```python
from build123d import *

# Parameters (mm, degrees)
F0_W      = 75
F0_H      = 75
F1_DEPTH  = 5
F3_DEPTH  = 40
F4_W      = 18
F4_H      = 17.9855290949
F4_W_2    = 12
F4_H_2    = 12
F4_H_3    = 18
F5_DEPTH  = 5
F6_DEPTH  = 15
F7_W      = 12
F7_H      = 15
F8_DEPTH  = 5
F9_W      = 12
F9_H      = 15
F10_DEPTH = 5


with BuildPart() as f1:
    # F0 (on Top) → F1 (new body)
    with BuildSketch(Plane.XY):
        Rectangle(F0_W, F0_H)
    extrude(amount=F1_DEPTH)

    # F2 (on face) → F3 (join)
    with BuildSketch(Plane.XY.offset(5)):
        Polygon((18.3847763109, 0), (0, 18.3847763109), (-18.3847763109, 0), (0, -18.3847763109), align=None)
        Polygon((-14.1421356237, 0), (0, 14.1421356237), (14.1421356237, 0), (0, -14.1421356237), align=None, mode=Mode.SUBTRACT)
    extrude(amount=F3_DEPTH)

    # F4 (on face) → F5 (join)
    with BuildSketch(Plane.XY.offset(5)):
        with Locations((0.0273990361, 28.5072354525)):
            Rectangle(F4_W, F4_H)
        with Locations((0.0273990361, 28.5144709051)):
            Rectangle(F4_W_2, F4_H_2, mode=Mode.SUBTRACT)
        with Locations((-28.5, 0)):
            Rectangle(F4_W, F4_H_3)
        with Locations((-28.5, 0)):
            Rectangle(F4_W_2, F4_H_2, mode=Mode.SUBTRACT)
    extrude(amount=F5_DEPTH)

    # F6 (add): faces of the model
    f6_faces = [f1.faces().sort_by_distance(p)[0] for p in [
        (8.772942899, 28.5072354525, 10),
        (-28.5, 8.7454415588, 10),
        (-28.5, 8.7454415588, 10),
    ]]
    extrude(f6_faces, amount=F6_DEPTH)

    # F7 (on face) → F8 (cut)
    with BuildSketch(Plane(origin=(-37.5, 0, 0), x_dir=(0, -1, 0), z_dir=(-1, 0, 0))):
        with Locations((0, 17.5)):
            Rectangle(F7_W, F7_H)
    extrude(amount=-F8_DEPTH, mode=Mode.SUBTRACT)

    # F9 (on face) → F10 (cut)
    with BuildSketch(Plane(origin=(0, 37.5, 0), x_dir=(-1, 0, 0), z_dir=(0, 1, 0))):
        with Locations((0, 17.5)):
            Rectangle(F9_W, F9_H)
    extrude(amount=-F10_DEPTH, mode=Mode.SUBTRACT)


solid = f1.part
```
Geometry check sheet. Reference: the model listing, model coordinates, mm. A direction names the side the tool comes from. Give positions to 0.01 mm unless a question says otherwise; leave off trailing zeros. Loops run counter-clockwise (first coordinate to the right, second up) from the corner with the lowest first, then second, coordinate; pieces in that order, holes last. Notation, with made-up numbers: M -21.75,71.5 L 20.25,71.5 A13 ccw 20.25,79.5 Z; hole C 50,-25.75 d4. An arc over 180 degrees is marked long. Write item = value, one per line.
(1) Release check for a two-part mould opening along X. For faces 6 (the face through (-30, 6, 15)), 7 (the face through (-8.973, 28, 15)), 8 (the face through (9.321, 9.064, 24.72)), 9 (the face through (7.17, -6.97, 24.72)) record: released by +X, released by -X, zero draft, split by the parting line, or undercut.
Answer below:
face_6 = undercut
face_7 = released by -X
face_8 = released by +X
face_9 = undercut
(2) Material ranges on line 1 (X direction, y = 1, z = 20.5); line 2 (Y direction, x = -27.5, z = 24.5); line 3 (X direction, y = -5.5, z = 15), recorded low to high. Write a range as [from, to].
Answer below:
line_1 = [-22.5, -19.5], [-17.38, -13.14], [13.14, 17.38]
line_2 = [-9, -6], [6, 9]
line_3 = [-22.5, -19.5], [-12.88, -8.64], [8.64, 12.88]
(3) Sectioned sample at D-D, the plane x = -20.5. Record the cut outline in (y, z).
Answer below:
outline = M -37.5,0 L 37.5,0 L 37.5,5 L 9,5 L 9,25 L -9,25 L -9,5 L -37.5,5 Z
(4) Sectioned sample at A-A, the plane z = 11. State how many separate pieces and enclosed holes the cut face has, plus the area to 3 significant figures.
Answer below:
separate_pieces = 3
enclosed_holes = 1
area = 564 mm2
(5) Gauge pin test, flat ends, axial feed: pin 1 Ø6 at (x, z) = (20, 27) entering from -Y; pin 2 Ø3 at (y, z) = (-7.5, 25.5) entering from +X; pin 3 Ø8 at (y, z) = (-14.5, 13) entering from -X; pin 4 Ø8 at (x, y) = (-25.5, 8.5) entering from -Z. Record the tip position at first contact, or that the pin passes through.
Answer below:
pin_1 = -1.38
pin_2 = 12.38
pin_3 = -7.88
pin_4 = 0
(6) Sectioned sample at B-B, the plane y = 30. Record the cut outline in (x, z), plus the area to 3 significant figures.
Answer below:
outline = M -37.5,0 L 37.5,0 L 37.5,5 L 9.03,5 L 9.03,25 L 6.03,25 L 6.03,5 L -5.97,5 L -5.97,25 L -8.97,25 L -8.97,5 L -37.5,5 Z
area = 495 mm2
(7) Sectioned sample at C-C, the plane z = 27.5. Record the cut outline in (x, y), plus the area to 3 significant figures.
Answer below:
outline = M -18.38,0 L 0,-18.38 L 18.38,0 L 0,18.38 Z; hole M -14.14,0 L 0,-14.14 L 14.14,0 L 0,14.14 Z
area = 276 mm2
(8) Tool access check on faces 1 (the face through (-7.17, 6.97, 24.72)), 2 (the face through (9.064, -9.321, 24.72)), 3 (the face through (-29, 9, 15)), 4 (the face through (6, 36, 17)), 5 (the face through (-21, 2, 25)). Record the directions out of +Z, -Z, +X, -X, +Y, -Y that give a thin tool (end or side, any length) a straight path to the whole face; none if there is none.
Answer below:
face_1 = +Z
face_2 = +Z, +X, -Y
face_3 = +Z, -X, +Y
face_4 = +Z, +Y
face_5 = +Z, -X, +Y, -Y
